Source: CAD feature listing. Evaluate the final solid. Frame: model axes, mm. Give positions to 0.01 mm unless a question says otherwise; leave off trailing zeros. Loops run counter-clockwise (first coordinate to the right, second up) from the corner with the lowest first, then second, coordinate; pieces in that order, holes last. Notation, with made-up numbers: M -10,3.25 L 3,3.25 A3 ccw 3,8.25 Z; hole C 50.25,-7.75 d4. An arc over 180 degrees is marked long. Answer in a Markdown table with one row per item.
```python
from build123d import *

# Parameters (mm, degrees)
BOARD_DEPTH = 1.6194


with BuildPart() as part:
    # Sketch1 → Board (new body)
    with BuildSketch(Plane.XY):
        with BuildLine():
            Line((10, 29), (10, 57.01299))
            ThreePointArc((10, 57.01299), (10.185190901, 57.290158106), (10.51213, 57.22513))
            ThreePointArc((10.51213, 57.22513), (12.777621512, 57.222368475), (12.77487, 59.48786))
            ThreePointArc((12.77487, 59.48786), (12.709829188, 59.814802566), (12.987, 60))
            Line((12.987, 60), (37.01299, 60))
            ThreePointArc((37.01299, 60), (37.290150019, 59.814804479), (37.22512, 59.48787))
            ThreePointArc((37.22512, 59.48787), (37.223732391, 57.223742391), (39.48786, 57.22513))
            ThreePointArc((39.48786, 57.22513), (39.814807186, 57.290168899), (40, 57.01299))
            Line((40, 57.01299), (40, 29))
            ThreePointArc((40, 29), (39.121323273, 26.878676727), (37, 26))
            Line((37, 26), (13, 26))
            ThreePointArc((13, 26), (10.878679656, 26.878679656), (10, 29))
        make_face()
    extrude(amount=BOARD_DEPTH)


solid = part.part
```
1) Pull-direction query (X, two-part tool) for faces 1 (the cylindrical face through (37.2, 57.25, 0.8)), 2 (the flat face through (10, 43, 1)), 3 (the cylindrical face through (12.752, 57.198, 0.798)), 4 (the flat face through (25, 26, 1)); classes: released by +X, released by -X, zero draft, split by the parting line, or undercut.
Reply:
| item | result |
|---|---|
| face 1 | undercut |
| face 2 | released by -X |
| face 3 | undercut |
| face 4 | zero draft |
2) Material intervals for L1, parallel to X at y = 58.5, z = 1.05; L2, parallel to Y at x = 11, z = 0.9; L3, parallel to Y at x = 38, z = 0.85, sorted ascending.
Reply:
| item | result |
|---|---|
| L1 | x = 13.24 to 36.76 |
| L2 | y = 26.76 to 56.89 |
| L3 | y = 26.17 to 56.8 |
3) Section A-A, the plane z = 0.95. Return loops of the section in (x, y), then the cut area to 3 significant figures.
Reply:
| item | result |
|---|---|
| outline | M 10,29 A3 ccw 13,26 L 37,26 A3 ccw 40,29 L 40,57.01 A0.3 ccw 39.49,57.23 A1.6 cw 37.23,59.49 A0.3 ccw 37.01,60 L 12.99,60 A0.3 ccw 12.77,59.49 A1.6 cw 10.51,57.23 A0.3 ccw 10,57.01 Z |
| area | 998 mm² |
